Geometry: final body of the model. Coordinates: model frame, mm. A direction names the side the tool comes from. Coordinates: 2 decimals unless noted, no trailing zeros. Order: outer loops, then holes, each group sorted by start corner. A loop starts at its lowest first (then second) coordinate and runs counter-clockwise, first axis right, second up. Notation, with made-up numbers: (-24, -32.5) - (-12, -32.5) arc R24 cw to (-12, -11.5) - close; hole circle Ø10 at (28, 87.5). An arc over 180 degrees is marked (long way). Use a Markdown table: item, result. Add a question column.
```python
from build123d import *

# Parameters (mm, degrees)
ESQUISSE1_W             = 3.5
ESQUISSE1_H             = 7
BOSS_EXTRU_1_DEPTH      = 3.5
ESQUISSE2_W             = 3
ESQUISSE2_H             = 3.5
ENL_V_MAT_EXTRU_1_DEPTH = 1
ESQUISSE3_W             = 3
ESQUISSE3_H             = 3.5
ENL_V_MAT_EXTRU_2_DEPTH = 1
ENL_V_MAT_EXTRU_4_DEPTH = 10


with BuildPart() as part:
    # Esquisse1 → Boss.-Extru.1 (new body)
    with BuildSketch(Plane.XY):
        with Locations((0.25, 0)):
            Rectangle(ESQUISSE1_W, ESQUISSE1_H)
    extrude(amount=BOSS_EXTRU_1_DEPTH)

    # Esquisse2 → Enlèv. mat.-Extru.1 (cut)
    with BuildSketch(Plane(origin=(0, 3.5, 0), x_dir=(1, 0, 0), z_dir=(0, 1, 0))):
        with Locations((0.25, -1.75)):
            Rectangle(ESQUISSE2_W, ESQUISSE2_H)
    extrude(amount=-ENL_V_MAT_EXTRU_1_DEPTH, mode=Mode.SUBTRACT)

    # Esquisse3 → Enlèv. mat.-Extru.2 (cut)
    with BuildSketch(Plane(origin=(0, -3.5, 0), x_dir=(-1, 0, 0), z_dir=(0, -1, 0))):
        with Locations((-0.25, -1.75)):
            Rectangle(ESQUISSE3_W, ESQUISSE3_H)
    extrude(amount=-ENL_V_MAT_EXTRU_2_DEPTH, mode=Mode.SUBTRACT)

    # Esquisse5 → Enlèv. mat.-Extru.4 (cut)
    with BuildSketch(Plane(origin=(2, 0, 0), x_dir=(0, 0, -1), z_dir=(1, 0, 0))):
        with BuildLine():
            Line((-3.5, -2), (-3.5, 2))
            ThreePointArc((-3.5, 2), (-1.5, 0), (-3.5, -2))
        make_face()
    extrude(amount=-ENL_V_MAT_EXTRU_4_DEPTH, mode=Mode.SUBTRACT)


solid = part.part
```
1) Ray query, line 1 along X through (y, z) = (-2.75, 2.4); line 2 along Y through (x, z) = (0.7, 0.2); line 3 along Y through (x, z) = (-0.05, 2.05). Return the intervals inside material, ascending.
2) Section C-C (z = 0.6). Return loops of the section in (x, y), then the cut area to 3 significant figures.
3) Section D-D (y = 0). Return loops of the section in (x, z), then the cut area to 3 significant figures.
4) Set-up query: faces 5 (the face through (0, 0, 0)), 6 (the face through (-1.25, 3, 2)), 7 (the face through (-1.25, -3, 2)). Return all of +Z, -Z, +X, -X, +Y, -Y with unobstructed straight access to the full face (end or side cutting, diameter ignored); none if empty.
5) Pin query (flat end, axial travel): pin 1 (0.9 mm diameter, centred on x = 0, z = 2.5, fed in from -Y). Return the tip coordinate at first contact, or that it passes through.
6) Section B-B (x = 0.15). Return loops of the section in (y, z), then the cut area to 3 significant figures.
7) Section A-A (z = 2.2). Return loops of the section in (x, y).
8) Draft query along X for faces 1 (the face through (0, 2.5, 2)), 2 (the face through (1.75, 3, 2)), 3 (the face through (-1.5, 0, 1)), 4 (the face through (0.2, 2.3, 3.5)). Return one class per face: pulls with the +X half, pulls with the -X half, needs draft (parallel to the pull), parting line crosses it, or undercut.
Values follow:
| question | item | result |
|---|---|---|
| 1 | line 1 | x = -1.5 to -1.25, 1.75 to 2 |
| 1 | line 2 | y = -2.5 to 2.5 |
| 1 | line 3 | y = -2.5 to -1.38, 1.38 to 2.5 |
| 2 | outline | (-1.5, -3.5) - (-1.25, -3.5) - (-1.25, -2.5) - (1.75, -2.5) - (1.75, -3.5) - (2, -3.5) - (2, 3.5) - (1.75, 3.5) - (1.75, 2.5) - (-1.25, 2.5) - (-1.25, 3.5) - (-1.5, 3.5) - close |
| 2 | area | 18.5 mm² |
| 3 | outline | (-1.5, 0) - (2, 0) - (2, 1.5) - (-1.5, 1.5) - close |
| 3 | area | 5.25 mm² |
| 4 | face 5 | -Z, +X, -X, +Y, -Y |
| 4 | face 6 | +Z, -Z, +Y |
| 4 | face 7 | +Z, -Z, -Y |
| 5 | pin 1 | stops at y = -2.5 |
| 6 | outline | (-2.5, 0) - (2.5, 0) - (2.5, 3.5) - (2, 3.5) arc R2 cw to (-2, 3.5) - (-2.5, 3.5) - close |
| 6 | area | 11.2 mm² |
| 7 | outline | (-1.5, -3.5) - (-1.25, -3.5) - (-1.25, -2.5) - (1.75, -2.5) - (1.75, -3.5) - (2, -3.5) - (2, -1.52) - (-1.5, -1.52) - close; (-1.5, 1.52) - (2, 1.52) - (2, 3.5) - (1.75, 3.5) - (1.75, 2.5) - (-1.25, 2.5) - (-1.25, 3.5) - (-1.5, 3.5) - close |
| 8 | face 1 | undercut |
| 8 | face 2 | undercut |
| 8 | face 3 | pulls with the -X half |
| 8 | face 4 | needs draft |
